from build123d import *

# Parameters (mm, degrees)
F1_DEPTH = 50
F2_W     = 22
F2_H     = 9.5
F3_DEPTH = 13.7632765638
F4_DEPTH = 0.4


with BuildPart() as f1:
    # F0 (on Front) → F1 (new body)
    with BuildSketch(Plane.XZ):
        Polygon((-0.0777817459, 0.0777817459), (0, 0), (13.6522765638, 13.6522765638), (68.0406461445, 13.6522765638), (81.6929227083, 0), (81.7835545517, 0.0649316484), (80.9242431001, 0.9242431001), (68.0862096363, 13.7622765638), (13.606713072, 13.7622765638), align=None)
    extrude(amount=F1_DEPTH)

    # F2 (on face) → F3 (cut, through all)
    with BuildSketch(Plane.XY.offset(13.7622765638)):
        with Locations((40.8464613542, -45.25)):
            Rectangle(F2_W, F2_H)
    extrude(amount=-F3_DEPTH, mode=Mode.SUBTRACT)

    # F4 (cut): a face of the model
    f4_faces = [f1.faces().sort_by_distance(p)[0] for p in [
        (40.8464613542, -40.5, 13.7072765638),
    ]]
    extrude(f4_faces, amount=-F4_DEPTH, mode=Mode.SUBTRACT)


solid = f1.part
Here's how the part is built. I have some questions about the finished solid (model axes, mm). Coordinates: 2 decimals unless noted, no trailing zeros. Loops run counter-clockwise (first coordinate to the right, second up) from the corner with the lowest first, then second, coordinate; pieces in that order, holes last.
1. Imagine slicing it at A-A, the plane y = -44.5. Please give me the cut outline in (x, z), and give its area (3 significant figures).
2. For P1, Ø15, axis at x = 32.5, y = -22, coming from the -Z side; P2, Ø8, axis at y = -42, z = 8.5, coming from the +X side; P3, Ø3, axis at x = 67.5, y = -38, coming from the -Z side, each with a flat end and sliding along its axis, tell me the tip position at first contact or that it passes through.
3. Imagine slicing it at B-B, the plane y = -18. Please give me the cut outline in (x, z).
4. Imagine slicing it at D-D, the plane x = 56.5. Please give me the cut outline in (y, z), and give its area (3 significant figures).
5. Imagine slicing it at C-C, the plane z = 10.5. Please give me the cut outline in (x, y), and give its area (3 significant figures).
6. I need wall thicknesses on L1, parallel to X at y = -10, z = 4.25; L2, parallel to X at y = -20.5, z = 7.75; L3, parallel to Z at x = 72, y = -45. Which ranges of each line are inside material? Lowest first, please.
Taken from the geometry:
1. outline: (-0.08, 0.08) - (0, 0) - (13.65, 13.65) - (29.85, 13.65) - (29.85, 13.76) - (13.61, 13.76) - close; (51.85, 13.65) - (68.04, 13.65) - (81.69, 0) - (81.78, 0.06) - (68.09, 13.76) - (51.85, 13.76) - close
1. area: 7.82 mm2
2. P1: stops at z = 13.65
2. P2: stops at x = 77.35
2. P3: stops at z = 12.69
3. outline: (-0.08, 0.08) - (0, 0) - (13.65, 13.65) - (68.04, 13.65) - (81.69, 0) - (81.78, 0.06) - (68.09, 13.76) - (13.61, 13.76) - close
4. outline: (-50, 13.65) - (0, 13.65) - (0, 13.76) - (-50, 13.76) - close
4. area: 5.50 mm2
5. outline: (10.34, -50) - (10.5, -50) - (10.5, 0) - (10.34, 0) - close; (71.19, -50) - (71.35, -50) - (71.35, 0) - (71.19, 0) - close
5. area: 15.6 mm2
6. L1: x = 4.09 to 4.25, 77.44 to 77.6
6. L2: x = 7.59 to 7.75, 73.94 to 74.1
6. L3: z = 9.69 to 9.85
